Here's how the part is built. I have some questions about the finished solid (model axes, mm). Round coordinates to 2 decimals unless told otherwise and drop trailing zeros. Write each loop counter-clockwise with the first axis right and the second up, starting at its lowest first coordinate (ties: lowest second). Pieces come first, ordered by that corner, then holes. Notation, with made-up numbers: (-26, 10.25) -> (30, 10.25) arc R10 ccw to (30, 16.25) -> close; hole circle Ø6 at (79, 73). An arc over 180 degrees is marked (long way). Answer as CSV lines item,"result".
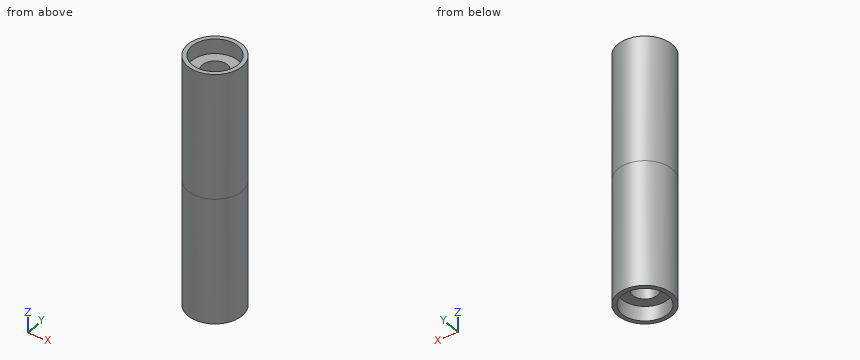
```python
from build123d import *

# Parameters (mm, degrees)
F0_R     = 13
F0_R_2   = 11
F0_R_3   = 6
F1_DEPTH = 60
F2_DEPTH = 7
F3_DEPTH = 15


with BuildPart() as f1:
    # F0 (on Top) → F1 (new body)
    with BuildSketch(Plane.XY):
        Circle(F0_R)
        Circle(F0_R_2, mode=Mode.SUBTRACT)
        Circle(F0_R_2)
        Circle(F0_R_3, mode=Mode.SUBTRACT)
        Circle(F0_R_3)
    extrude(amount=F1_DEPTH)

    # F0 (on Top) → F2 (cut)
    with BuildSketch(Plane.XY):
        Circle(F0_R_2)
        Circle(F0_R_3, mode=Mode.SUBTRACT)
        Circle(F0_R_3)
    extrude(amount=F2_DEPTH, mode=Mode.SUBTRACT)

    # F0 (on Top) → F3 (cut)
    with BuildSketch(Plane.XY):
        Circle(F0_R_3)
    extrude(amount=F3_DEPTH, mode=Mode.SUBTRACT)

    # F5: F1 across plane


with BuildPart() as f1_1:
    add(f1.part)
    add(f1.part.mirror(Plane.XY.offset(60)))


solid = f1_1.part
```
1. If I drill on line 1 (Y direction, x = 0, z = 5.5); line 2 (Y direction, x = 0, z = 107.5); line 3 (Z direction, x = 10, y = -4.5), over which ranges is the centre line in solid material (lowest first)?
Numbers:
line 1,"y = -13 to -11, 11 to 13"
line 2,"y = -13 to -6, 6 to 13"
line 3,"z = 7 to 113"
2. Suppose I cut it at D-D on x = 9.25. Please give me the cut outline in (y, z).
Numbers:
outline,"(-9.13, 0) -> (-5.95, 0) -> (-5.95, 7) -> (5.95, 7) -> (5.95, 0) -> (9.13, 0) -> (9.13, 120) -> (5.95, 120) -> (5.95, 113) -> (-5.95, 113) -> (-5.95, 120) -> (-9.13, 120) -> close"
3. Suppose I cut it at C-C on z = 54.5. Please give me the cut outline in (x, y).
Numbers:
outline,"circle Ø26 at (0, 0)"
4. Suppose I cut it at A-A on y = 0. Please give me the cut outline in (x, z), and give its area (3 significant figures).
Numbers:
outline,"(-13, 0) -> (-11, 0) -> (-11, 7) -> (-6, 7) -> (-6, 15) -> (6, 15) -> (6, 7) -> (11, 7) -> (11, 0) -> (13, 0) -> (13, 120) -> (11, 120) -> (11, 113) -> (6, 113) -> (6, 105) -> (-6, 105) -> (-6, 113) -> (-11, 113) -> (-11, 120) -> (-13, 120) -> close"
area,"2,620 mm^2"
5. For pin 1 Ø10 at (x, y) = (-2.5, 3) entering from -Z; pin 2 Ø11 at (x, y) = (0, 0) entering from +Z; pin 3 Ø9.5 at (x, y) = (-1.5, -1) entering from +Z, each with a flat end and sliding along its axis, tell me the tip position at first contact or that it passes through.
Numbers:
pin 1,"stops at z = 7"
pin 2,"stops at z = 105"
pin 3,"stops at z = 113"
